from build123d import *

# Parameters (mm, degrees)
F1_DEPTH      = 12.7
F3_DEPTH      = 28.575
F5_D          = 3.175
F6_D          = 3.175
F7_R          = 19.05
F8_DEPTH      = 46.99
F8_DEPTH_BACK = 44.196
F9_R          = 1.524
F10_R         = 1.524


with BuildPart() as f1:
    # F0 (on Top) → F1 (new body)
    with BuildSketch(Plane.XY):
        with BuildLine():
            ThreePointArc((29.1204104367, 19.05), (34.798, 0), (29.1204104367, -19.05))
            Line((29.1204104367, -19.05), (31.75, -19.05))
            Line((31.75, -19.05), (34.925, -19.05))
            ThreePointArc((34.925, -19.05), (37.1700640303, -19.9799359697), (38.1, -22.225))
            Line((38.1, -22.225), (38.1, -25.4))
            Line((38.1, -25.4), (38.1, -36.5125))
            ThreePointArc((38.1, -36.5125), (38.5649679849, -37.6350320151), (39.6875, -38.1))
            Line((39.6875, -38.1), (47.625, -38.1))
            Line((47.625, -38.1), (47.625, 38.1))
            Line((47.625, 38.1), (39.6875, 38.1))
            ThreePointArc((39.6875, 38.1), (38.5649679849, 37.6350320151), (38.1, 36.5125))
            Line((38.1, 36.5125), (38.1, 25.4))
            Line((38.1, 25.4), (38.1, 22.225))
            ThreePointArc((38.1, 22.225), (37.1700640303, 19.9799359697), (34.925, 19.05))
            Line((34.925, 19.05), (31.75, 19.05))
            Line((31.75, 19.05), (29.1204104367, 19.05))
        make_face()
    extrude(amount=F1_DEPTH)

    # F2 (on Top) → F3 (join)
    with BuildSketch(Plane.XY):
        with BuildLine():
            ThreePointArc((26.1160885863, 18.0558139377), (31.75, 0), (26.1160885863, -18.0558139377))
            ThreePointArc((26.1160885863, -18.0558139377), (26.0761118369, -18.7105456091), (26.6373982331, -19.05))
            Line((26.6373982331, -19.05), (29.1204104367, -19.05))
            ThreePointArc((29.1204104367, -19.05), (34.798, 0), (29.1204104367, 19.05))
            Line((29.1204104367, 19.05), (26.6373982331, 19.05))
            ThreePointArc((26.6373982331, 19.05), (26.0761118369, 18.7105456091), (26.1160885863, 18.0558139377))
        make_face()
    extrude(amount=F3_DEPTH)

    # F5 (through all)
    with Locations(Plane(origin=(0, 0, 0), x_dir=(0, 1, 0), z_dir=(-1, 0, 0))):
        with Locations((-29.21, -6.35)):
            Hole(F5_D / 2)

    # F6 (through all)
    with Locations(Plane(origin=(0, 0, 0), x_dir=(0, 1, 0), z_dir=(-1, 0, 0))):
        with Locations((29.21, -6.35)):
            Hole(F6_D / 2)

    # F7 (on Front) → F8 (cut, two sides)
    with BuildSketch(Plane.XZ) as f8_sk:
        with Locations((65.659, 6.35)):
            Circle(F7_R)
    extrude(amount=F8_DEPTH, mode=Mode.SUBTRACT)
    extrude(f8_sk.sketch, amount=-F8_DEPTH_BACK, mode=Mode.SUBTRACT)

    # F9
    f9_edges = [f1.edges().sort_by_distance(p)[0] for p in [
        (29.12041, 19.05, 20.6375),
    ]]
    fillet(f9_edges, radius=F9_R)

    # F10
    f10_edges = [f1.edges().sort_by_distance(p)[0] for p in [
        (29.12041, -19.05, 20.6375),
    ]]
    fillet(f10_edges, radius=F10_R)


solid = f1.part
Model file for the job. Use its own axes, mm. A direction names the side the tool comes from. Coordinates: 2 decimals unless noted, no trailing zeros. Order: outer loops, then holes, each group sorted by start corner. A loop starts at its lowest first (then second) coordinate and runs counter-clockwise, first axis right, second up. Notation, with made-up numbers: (34, 28.5) -> (64, 28.5) arc R22 ccw to (64, 53.5) -> close; hole circle Ø9 at (58, -2). An arc over 180 degrees is marked (long way). Return JSON: item names as keys, results as strings. Group by question number.
Item 1: Pull direction Z, two halves, no side cores. Call faces 4 (the cylindrical face through (46.61, 0.53, 6.44)), 5 (the flat face through (39, 1, 0)), 6 (the flat face through (44, -38.1, 6)): pulls with the +Z half, pulls with the -Z half, needs draft (parallel to the pull), parting line crosses it, or undercut.
Item 2: Flat gauge pins, fed straight in: P1, Ø4, axis at y = -30.5, z = 7.5, coming from the -X side; P2, Ø3, axis at y = -23.5, z = 4.5, coming from the +X side; P3, Ø8, axis at x = 42, y = 30.5, coming from the +Z side; P4, Ø1.5, axis at x = 28.5, y = 13.5, coming from the -Z side. Where does each tip first touch, or does it go through?
Item 3: Saw through at D-D on z = 14. Write the cut outline in (x, y), then the cut area to 3 significant figures.
Item 4: Wall check: line 1 along Y through (x, z) = (42.5, 6.35); line 2 along Z through (x, y) = (44, 29.21); line 3 along X through (y, z) = (-22, 6.5). Give the ranges that are in metal, low to high. Write a range as [from, to].
Item 5: Tool access for faces 1 (the flat face through (30, -19.05, 8)), 2 (the flat face through (38.1, 31, 6)), 3 (the cylindrical face through (29.02, -18.86, 20.75)): list every direction of +Z, -Z, +X, -X, +Y, -Y with a clear straight run to the whole face (end or side of a thin tool).
Item 6: Saw through at A-A on z = 6.35. State how many separate pieces and enclosed holes the cut face has, then the cut area to 3 significant figures.
Values found:
{
 "1": {"face 4": "undercut", "face 5": "pulls with the -Z half", "face 6": "needs draft"},
 "2": {"P1": "stops at x = 38.1", "P2": "stops at x = 46.91", "P3": "stops at z = 12.7", "P4": "stops at z = 0"},
 "3": {"outline": "(26.12, -18.06) arc R0.63 ccw to (26.64, -19.05) -> (28.28, -19.05) arc R1.52 ccw to (29.58, -18.33) arc R34.8 ccw to (29.58, 18.33) arc R1.52 ccw to (28.28, 19.05) -> (26.64, 19.05) arc R0.63 ccw to (26.12, 18.06) arc R31.75 cw to start", "area": "123 mm2"},
 "4": {"line 1": "y = [-38.1, -30.8], [-27.62, 27.62], [30.8, 38.1]", "line 2": "z = [0, 4.76], [7.94, 12.7]", "line 3": "x = [38.09, 46.61]"},
 "5": {"face 1": "+Z, -Z, -X, -Y", "face 2": "+Z, -Z, -X, +Y", "face 3": "+Z, +X, -Y"},
 "6": {"separate pieces": "3", "enclosed holes": "0", "area": "916 mm2"}
}
